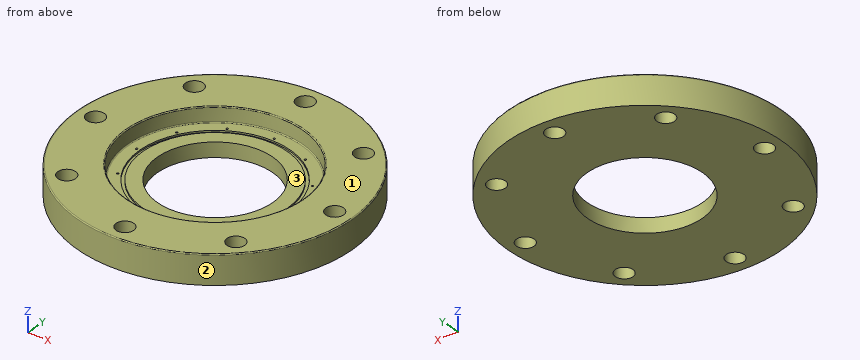
from build123d import *

# Parameters (mm, degrees)
SKETCH1_R          = 171.45
EXTRUDE1_DEPTH     = 36.5125
SKETCH2_R          = 11.1125
EXTRUDE2_DEPTH     = 37.5125
CIRPATTERN1_COUNT  = 8
FILLET1_R          = 1.154545455
SKETCH4_R          = 72
CUT_EXTRUDE1_DEPTH = 120
CIRPATTERN2_COUNT  = 12
SKETCH5_R          = 94
SKETCH5_R_2        = 90
CUT_EXTRUDE2_DEPTH = 2


with BuildPart() as part:
    # Sketch1 → Extrude1 (new body)
    with BuildSketch(Plane.XY):
        Circle(SKETCH1_R)
    extrude(amount=EXTRUDE1_DEPTH)

    # Sketch2 → Extrude2 (cut, through all)
    with BuildSketch(Plane.XY.offset(36.5125)):
        with Locations((0, 149.225)):
            Circle(SKETCH2_R)
    extrude2 = extrude(amount=-EXTRUDE2_DEPTH, mode=Mode.SUBTRACT)

    # CirPattern1: Extrude2 ×8 about axis
    cirpattern1_axis = Axis((0, 0, 0), (0, 0, 1))
    for i in range(1, CIRPATTERN1_COUNT):
        add(extrude2.rotate(cirpattern1_axis, i * 360 / CIRPATTERN1_COUNT), mode=Mode.SUBTRACT)

    # Sketch3 → Cut-Revolve1 (revolve, cut)
    with BuildSketch(Plane(origin=(0, 0, 0), x_dir=(0, 0, -1), z_dir=(1, 0, 0))):
        Polygon((-36.5125, 109.9185), (-18.25625, 109.347), (-18.25625, 0), (-36.5125, 0), align=None)
    revolve(axis=Axis((0, 0, 18.25625), (0, 0, 1)), mode=Mode.SUBTRACT)

    # Fillet1
    fillet1_edges = [part.edges().sort_by_distance(p)[0] for p in [
        (0, -109.347, 18.25625),
        (0, -109.9185, 36.5125),
        (-171.45, 0, 36.5125),
    ]]
    fillet(fillet1_edges, radius=FILLET1_R)

    # Sketch4 → Cut-Extrude1 (cut)
    with BuildSketch(Plane(origin=(0, 0, 0), x_dir=(-1, 0, 0), z_dir=(0, 0, -1))):
        Circle(SKETCH4_R)
    extrude(amount=-CUT_EXTRUDE1_DEPTH, mode=Mode.SUBTRACT)

    # Sketch8 → M3x0.5 Tapped Hole1 (revolve, cut)
    with BuildSketch(Plane(origin=(0, 97.79, 18.25625), x_dir=(0, -1, 0), z_dir=(1, 0, 0))):
        Polygon((0, 0), (0, 12.751075774), (1.25, 12), (1.25, 0), align=None)
    m3x0_5_tapped_hole1 = revolve(axis=Axis((0, 97.79, 24.60625), (0, 0, -1)), mode=Mode.SUBTRACT)

    # CirPattern2: M3x0.5 Tapped Hole1 ×12 about axis
    cirpattern2_axis = Axis((0, 0, 0), (0, 0, 1))
    for i in range(1, CIRPATTERN2_COUNT):
        add(m3x0_5_tapped_hole1.rotate(cirpattern2_axis, i * 360 / CIRPATTERN2_COUNT), mode=Mode.SUBTRACT)

    # Sketch5 → Cut-Extrude2 (cut)
    with BuildSketch(Plane(origin=(0, 0, 18.25625), x_dir=(-1, 0, 0), z_dir=(0, 0, -1))):
        Circle(SKETCH5_R)
        Circle(SKETCH5_R_2, mode=Mode.SUBTRACT)
    extrude(amount=CUT_EXTRUDE2_DEPTH, mode=Mode.SUBTRACT)


solid = part.part
Geometry: final body of the model. Coordinates: model frame, mm. Face numbers are marked on the shaded views. Give positions to 0.01 mm unless a question says otherwise; leave off trailing zeros. Answer as a JSON object with one key per item and string values.
Q1. Draft query along X for the marked faces 1, 2 and 3. Return one class per face: released by +X, released by -X, zero draft, split by the parting line, or undercut.
Entries:
{"face 1": "zero draft", "face 2": "split by the parting line", "face 3": "undercut"}
Q2. First-contact query: pin 1 (2 mm diameter, centred on x = 128.5, z = 30, fed in from -Y); pin 2 (3 mm diameter, centred on y = 39.5, z = 18.5, fed in from +X); pin 3 (8 mm diameter, centred on x = 54.5, y = 82.5, fed in from +Z). Flat tips, straight axial feed; report the tip coordinate or a pass-through.
Entries:
{"pin 1": "stops at y = -114.62", "pin 2": "stops at x = 167.19", "pin 3": "stops at z = 18.26"}
Q3. Material intervals for probe 1 along Y at (x, z) = (0, 13); probe 2 along Y at (x, z) = (-5, 25.5); probe 3 along X at (y, z) = (110.5, 21.5), sorted ascending.
Entries:
{"probe 1": "y = -171.45 to -160.34, -138.11 to -99.04, -96.54 to -72, 72 to 96.54, 99.04 to 138.11, 160.34 to 171.45", "probe 2": "y = -171.38 to -159.15, -139.3 to -109.46, 109.46 to 139.3, 159.15 to 171.38", "probe 3": "x = -131.09 to -115.45, -95.58 to 95.58, 115.45 to 131.09"}
Q4. Section A-A (z = 11.5). State how many separate pieces and enclosed holes the cut face has, plus the area to 3 significant figures.
Entries:
{"separate pieces": "1", "enclosed holes": "21", "area": "72,900 mm^2"}
